Design review of the part shown in the three views and the two pictorial views. Dimensions are in mm from the part's minimum x, y and z. Round coordinates to 2 decimals unless told otherwise and drop trailing zeros. Loops run counter-clockwise (first coordinate to the right, second up) from the corner with the lowest first, then second, coordinate; pieces in that order, holes last. Notation, with made-up numbers: (32.25, 64) -> (70.25, 64) arc R34 cw to (70.25, 97) -> close; hole circle Ø6 at (40, -13). An arc over 180 degrees is marked (long way). Write each question's results on one line, items separated by ' | '. Start each with the question number.
Item 1: We need section B-B (x = 400.5). Give the boundary of the cut face in (y, z), and give its area (3 significant figures).
Item 2: We need section A-A (z = 2.3). Give the number of separate pieces and of enclosed holes in the cut face, and give its area (3 significant figures).
Item 3: For L1, parallel to X at y = 46.5, z = 0.8; L2, parallel to X at y = 54, z = 2.35; L3, parallel to Y at x = 107, z = 0.3, list the stretches that pass through material, from the lowest coordinate up. Write a range as from..to.
Item 4: Clearance check with flat-ended pins moving along their axes: pin 1 Ø1.8 at (x, z) = (1.5, 2.5) entering from +Y; pin 2 Ø2 at (y, z) = (7.5, 1.5) entering from -X; pin 3 Ø3 at (x, z) = (596.5, 3.5) entering from -Y. State where each tip first meets the part, or that it passes through.
Item 5: We need section C-C (y = 65). Give the boundary of the cut face in (x, z).
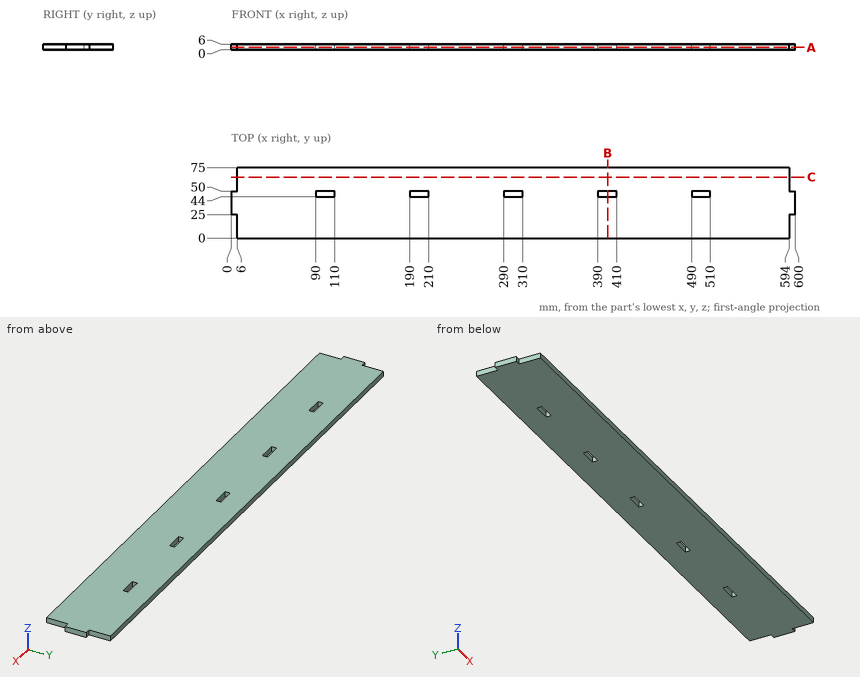
Here are the results:
1) outline: (0, 0) -> (44, 0) -> (44, 6) -> (0, 6) -> close; (50, 0) -> (75, 0) -> (75, 6) -> (50, 6) -> close | area: 414 mm2
2) separate pieces: 1 | enclosed holes: 5 | area: 43,800 mm2
3) L1: x = 0..90, 110..190, 210..290, 310..390, 410..490, 510..600 | L2: x = 6..594 | L3: y = 0..44, 50..75
4) pin 1: stops at y = 50 | pin 2: stops at x = 6 | pin 3: stops at y = 25
5) outline: (6, 0) -> (594, 0) -> (594, 6) -> (6, 6) -> close
